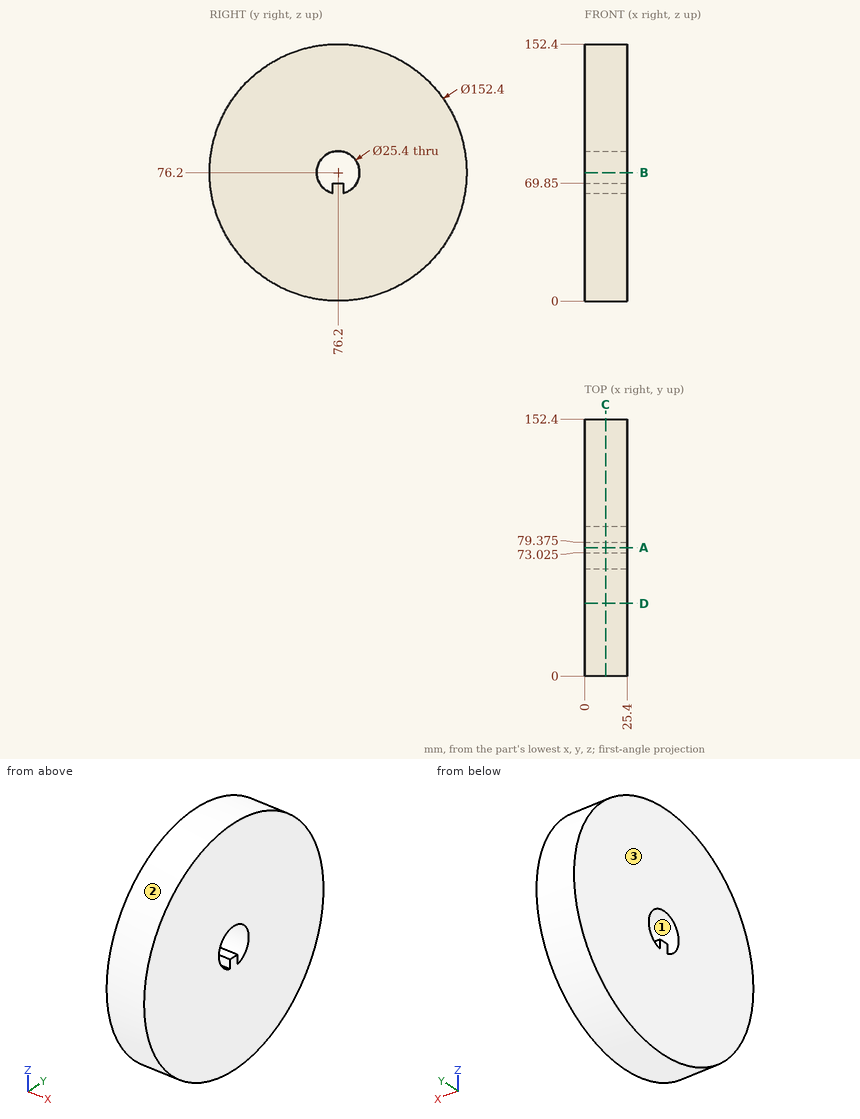
Here's the drawing with two shaded views (mm, measured from the low corner). I have some questions. Coordinates: 2 decimals unless noted, no trailing zeros. Write each loop counter-clockwise with the first axis right and the second up, starting at its lowest first coordinate (ties: lowest second). Pieces come first, ordered by that corner, then holes. Notation, with made-up numbers: M 14,-32 L 61,-32 A18 ccw 61,-11 Z; hole C 64,4 d5. An arc over 180 degrees is marked long. Write item = value, one per line. Start each with the question number.
Q1. If we section it at C-C, the plane x = 12.5: Write out the boundary of the cut face in (y, z) (3 decimals).
Q2. If we section it at B-B, the plane z = 76.2: Write out the boundary of the cut face in (x, y), then the cut area to 3 significant figures.
Q3. If we section it at A-A, the plane y = 76.2: Write out the boundary of the cut face in (x, z), then the cut area to 3 significant figures.
Q4. If we section it at D-D, the plane y = 43: Write out the boundary of the cut face in (x, z).
Q5. Thinking about a two-plate mould opening in Z: for the marked faces 1, 2 and 3, which applies, released by +Z, released by -Z, zero draft, split by the parting line, or undercut?
Q6. If I drill on L1, parallel to Z at x = 17.75, y = 76.2; L2, parallel to Y at x = 20, z = 36; L3, parallel to Z at x = 15.75, y = 123, over which ranges is the centre line in solid material (lowest first)? Write a range as [from, to].
Q7. I'm going to push flat-ended pins straight in: pin 1 (3 mm diameter, centred on x = 13, z = 66.5, fed in from +Y); pin 2 (1 mm diameter, centred on x = 10, y = 86.5, fed in from -Z); pin 3 (4 mm diameter, centred on x = 7.5, y = 45, fed in from +Z). Where does each tip first touch, or does it pass through?
Check sheet entries:
q1.outline = C 76.2,76.2 d152.4; hole M 73.025,63.903 L 73.025,69.85 L 79.375,69.85 L 79.375,63.903 A12.7 ccw long Z
q2.outline = M 0,0 L 25.4,0 L 25.4,63.5 L 0,63.5 Z; M 0,88.9 L 25.4,88.9 L 25.4,152.4 L 0,152.4 Z
q2.area = 3,230 mm²
q3.outline = M 0,0 L 25.4,0 L 25.4,69.85 L 0,69.85 Z; M 0,88.9 L 25.4,88.9 L 25.4,152.4 L 0,152.4 Z
q3.area = 3,390 mm²
q4.outline = M 0,7.61 L 25.4,7.61 L 25.4,144.79 L 0,144.79 Z
q5.face_1 = undercut
q5.face_2 = split by the parting line
q5.face_3 = zero draft
q6.L1 = [0, 69.85], [88.9, 152.4]
q6.L2 = [11.47, 140.93]
q6.L3 = [16.07, 136.33]
q7.pin_1 = 151.96
q7.pin_2 = 0.63
q7.pin_3 = 146.58
